from build123d import *

# Parameters (mm, degrees)
F0_W         = 12.7
F0_H         = 12.7
F1_DEPTH     = 12.7
F2_T1_DEPTH  = 6.35
F2_T3_DEPTH  = 6.35
F2_T5_DEPTH  = 6.35
F2_S9_W      = 3.175
F2_S9_H      = 3.175
F2_T10_DEPTH = 3.175
F2_S15_W     = 3.175
F2_S15_H     = 3.175
F2_T16_DEPTH = 3.175
F2_S21_W     = 3.175
F2_S21_H     = 3.175
F2_T22_DEPTH = 3.175
F2_S27_W     = 3.175
F2_S27_H     = 3.175
F2_T28_DEPTH = 3.175
F2_S33_W     = 3.175
F2_S33_H     = 3.175
F2_T34_DEPTH = 3.175
F2_S39_W     = 3.175
F2_S39_H     = 3.175
F2_T40_DEPTH = 3.175
F2_S45_W     = 3.175
F2_S45_H     = 3.175
F2_T46_DEPTH = 3.175
F2_S51_W     = 3.175
F2_S51_H     = 3.175
F2_T52_DEPTH = 3.175
F3_R         = 0.79375
F4_DEPTH     = 6.2992


# Not quite as in the source:
# - a fillet or chamfer that OpenCascade refuses, or shapes differently, is made with other operations: its cross-section is extruded or revolved along the edge and cut away or added


with BuildPart() as f1:
    # F0 (on Top) → F1 (new body)
    with BuildSketch(Plane.XY):
        Rectangle(F0_W, F0_H)
        with BuildLine():
            ThreePointArc((-2.54, 1.905), (0, 3.175), (2.54, 1.905))
            Line((2.54, 1.905), (3.96875, 0))
            Line((3.96875, 0), (2.54, -1.905))
            ThreePointArc((2.54, -1.905), (0, -3.175), (-2.54, -1.905))
            Line((-2.54, -1.905), (-3.96875, 0))
            Line((-3.96875, 0), (-2.54, 1.905))
        make_face(mode=Mode.SUBTRACT)
    extrude(amount=F1_DEPTH)

    # F2: fillet of radius 3.175 on 12 edges, made by hand

    # F2_s2 → F2_t1 (cut)
    with BuildSketch(Plane.XY.offset(3.175)):
        with BuildLine():
            ThreePointArc((6.35, -3.175), (5.4200640303, -5.4200640303), (3.175, -6.35))
            Line((3.175, -6.35), (6.35, -6.35))
            Line((6.35, -6.35), (6.35, -3.175))
        make_face()
        with BuildLine():
            ThreePointArc((6.35, 3.175), (5.4200640303, 5.4200640303), (3.175, 6.35))
            Line((3.175, 6.35), (6.35, 6.35))
            Line((6.35, 6.35), (6.35, 3.175))
        make_face()
        with BuildLine():
            ThreePointArc((-3.175, 6.35), (-5.4200640303, 5.4200640303), (-6.35, 3.175))
            Line((-6.35, 3.175), (-6.35, 6.35))
            Line((-6.35, 6.35), (-3.175, 6.35))
        make_face()
        with BuildLine():
            ThreePointArc((-6.35, -3.175), (-5.4200640303, -5.4200640303), (-3.175, -6.35))
            Line((-3.175, -6.35), (-6.35, -6.35))
            Line((-6.35, -6.35), (-6.35, -3.175))
        make_face()
    extrude(amount=F2_T1_DEPTH, mode=Mode.SUBTRACT)

    # F2_s4 → F2_t3 (cut)
    with BuildSketch(Plane.YZ.offset(-3.175)):
        with BuildLine():
            ThreePointArc((-6.35, 9.525), (-5.4200640303, 11.7700640303), (-3.175, 12.7))
            Line((-3.175, 12.7), (-6.35, 12.7))
            Line((-6.35, 12.7), (-6.35, 9.525))
        make_face()
        with BuildLine():
            ThreePointArc((-6.35, 3.175), (-5.4200640303, 0.9299359697), (-3.175, 0))
            Line((-3.175, 0), (-6.35, 0))
            Line((-6.35, 0), (-6.35, 3.175))
        make_face()
        with BuildLine():
            ThreePointArc((6.35, 3.175), (5.4200640303, 0.9299359697), (3.175, 0))
            Line((3.175, 0), (6.35, 0))
            Line((6.35, 0), (6.35, 3.175))
        make_face()
        with BuildLine():
            ThreePointArc((6.35, 9.525), (5.4200640303, 11.7700640303), (3.175, 12.7))
            Line((3.175, 12.7), (6.35, 12.7))
            Line((6.35, 12.7), (6.35, 9.525))
        make_face()
    extrude(amount=F2_T3_DEPTH, mode=Mode.SUBTRACT)

    # F2_s6 → F2_t5 (cut)
    with BuildSketch(Plane.XZ.offset(-3.175)):
        with BuildLine():
            ThreePointArc((6.35, 9.525), (5.4200640303, 11.7700640303), (3.175, 12.7))
            Line((3.175, 12.7), (6.35, 12.7))
            Line((6.35, 12.7), (6.35, 9.525))
        make_face()
        with BuildLine():
            ThreePointArc((6.35, 3.175), (5.4200640303, 0.9299359697), (3.175, 0))
            Line((3.175, 0), (6.35, 0))
            Line((6.35, 0), (6.35, 3.175))
        make_face()
        with BuildLine():
            ThreePointArc((-6.35, 3.175), (-5.4200640303, 0.9299359697), (-3.175, 0))
            Line((-3.175, 0), (-6.35, 0))
            Line((-6.35, 0), (-6.35, 3.175))
        make_face()
        with BuildLine():
            ThreePointArc((-6.35, 9.525), (-5.4200640303, 11.7700640303), (-3.175, 12.7))
            Line((-3.175, 12.7), (-6.35, 12.7))
            Line((-6.35, 12.7), (-6.35, 9.525))
        make_face()
    extrude(amount=F2_T5_DEPTH, mode=Mode.SUBTRACT)


with BuildPart() as f2_tool8:
    # F2_s9 → F2_t10 (new body)
    with BuildSketch(Plane.YZ.offset(3.175)):
        with Locations((-4.7625, 1.5875)):
            Rectangle(F2_S9_W, F2_S9_H)
    extrude(amount=F2_T10_DEPTH)

    # F2_s11 → F2_t12 (revolve, cut)
    with BuildSketch(Plane(origin=(3.175, -3.175, 3.175), x_dir=(0, 0.7071067812, 0.7071067812), z_dir=(0, 0.7071067812, -0.7071067812))):
        with BuildLine():
            ThreePointArc((0, -3.175), (3.175, 0), (0, 3.175))
            Line((0, 3.175), (0, -3.175))
        make_face()
    revolve(axis=Axis((3.175, -3.175, 3.175), (1, 0, 0)), mode=Mode.SUBTRACT)


with BuildPart() as f1_1:
    add(f1.part)

    # F2_t7: cut F2_tool8
    add(f2_tool8.part, mode=Mode.SUBTRACT)


with BuildPart() as f2_tool14:
    # F2_s15 → F2_t16 (new body)
    with BuildSketch(Plane.YZ.offset(3.175)):
        with Locations((-4.7625, 11.1125)):
            Rectangle(F2_S15_W, F2_S15_H)
    extrude(amount=F2_T16_DEPTH)

    # F2_s17 → F2_t18 (revolve, cut)
    with BuildSketch(Plane(origin=(3.175, -3.175, 9.525), x_dir=(0, 0.7071067812, -0.7071067812), z_dir=(0, -0.7071067812, -0.7071067812))):
        with BuildLine():
            ThreePointArc((0, -3.175), (3.175, 0), (0, 3.175))
            Line((0, 3.175), (0, -3.175))
        make_face()
    revolve(axis=Axis((3.175, -3.175, 9.525), (1, 0, 0)), mode=Mode.SUBTRACT)


with BuildPart() as f1_2:
    add(f1_1.part)

    # F2_t13: cut F2_tool14
    add(f2_tool14.part, mode=Mode.SUBTRACT)


with BuildPart() as f2_tool20:
    # F2_s21 → F2_t22 (new body)
    with BuildSketch(Plane.XY.offset(9.525)):
        with Locations((-4.7625, -4.7625)):
            Rectangle(F2_S21_W, F2_S21_H)
    extrude(amount=F2_T22_DEPTH)

    # F2_s23 → F2_t24 (revolve, cut)
    with BuildSketch(Plane(origin=(-3.175, -3.175, 9.525), x_dir=(0.7071067812, 0.7071067812, 0), z_dir=(0.7071067812, -0.7071067812, 0))):
        with BuildLine():
            ThreePointArc((0, -3.175), (3.175, 0), (0, 3.175))
            Line((0, 3.175), (0, -3.175))
        make_face()
    revolve(axis=Axis((-3.175, -3.175, 9.525), (0, 0, 1)), mode=Mode.SUBTRACT)


with BuildPart() as f1_3:
    add(f1_2.part)

    # F2_t19: cut F2_tool20
    add(f2_tool20.part, mode=Mode.SUBTRACT)


with BuildPart() as f2_tool26:
    # F2_s27 → F2_t28 (new body)
    with BuildSketch(Plane.YZ.offset(3.175)):
        with Locations((4.7625, 11.1125)):
            Rectangle(F2_S27_W, F2_S27_H)
    extrude(amount=F2_T28_DEPTH)

    # F2_s29 → F2_t30 (revolve, cut)
    with BuildSketch(Plane(origin=(3.175, 3.175, 9.525), x_dir=(0, -0.7071067812, -0.7071067812), z_dir=(0, -0.7071067812, 0.7071067812))):
        with BuildLine():
            ThreePointArc((0, -3.175), (3.175, 0), (0, 3.175))
            Line((0, 3.175), (0, -3.175))
        make_face()
    revolve(axis=Axis((3.175, 3.175, 9.525), (1, 0, 0)), mode=Mode.SUBTRACT)


with BuildPart() as f1_4:
    add(f1_3.part)

    # F2_t25: cut F2_tool26
    add(f2_tool26.part, mode=Mode.SUBTRACT)


with BuildPart() as f2_tool32:
    # F2_s33 → F2_t34 (new body)
    with BuildSketch(Plane.YZ.offset(3.175)):
        with Locations((4.7625, 1.5875)):
            Rectangle(F2_S33_W, F2_S33_H)
    extrude(amount=F2_T34_DEPTH)

    # F2_s35 → F2_t36 (revolve, cut)
    with BuildSketch(Plane(origin=(3.175, 3.175, 3.175), x_dir=(0, -0.7071067812, 0.7071067812), z_dir=(0, 0.7071067812, 0.7071067812))):
        with BuildLine():
            ThreePointArc((0, -3.175), (3.175, 0), (0, 3.175))
            Line((0, 3.175), (0, -3.175))
        make_face()
    revolve(axis=Axis((3.175, 3.175, 3.175), (1, 0, 0)), mode=Mode.SUBTRACT)


with BuildPart() as f1_5:
    add(f1_4.part)

    # F2_t31: cut F2_tool32
    add(f2_tool32.part, mode=Mode.SUBTRACT)


with BuildPart() as f2_tool38:
    # F2_s39 → F2_t40 (new body)
    with BuildSketch(Plane.YZ.offset(-3.175)):
        with Locations((-4.7625, 1.5875)):
            Rectangle(F2_S39_W, F2_S39_H)
    extrude(amount=-F2_T40_DEPTH)

    # F2_s41 → F2_t42 (revolve, cut)
    with BuildSketch(Plane(origin=(-3.175, -3.175, 3.175), x_dir=(0, 0.7071067812, 0.7071067812), z_dir=(0, -0.7071067812, 0.7071067812))):
        with BuildLine():
            ThreePointArc((0, -3.175), (3.175, 0), (0, 3.175))
            Line((0, 3.175), (0, -3.175))
        make_face()
    revolve(axis=Axis((-3.175, -3.175, 3.175), (-1, 0, 0)), mode=Mode.SUBTRACT)


with BuildPart() as f1_6:
    add(f1_5.part)

    # F2_t37: cut F2_tool38
    add(f2_tool38.part, mode=Mode.SUBTRACT)


with BuildPart() as f2_tool44:
    # F2_s45 → F2_t46 (new body)
    with BuildSketch(Plane.XZ.offset(-3.175)):
        with Locations((-4.7625, 1.5875)):
            Rectangle(F2_S45_W, F2_S45_H)
    extrude(amount=-F2_T46_DEPTH)

    # F2_s47 → F2_t48 (revolve, cut)
    with BuildSketch(Plane(origin=(-3.175, 3.175, 3.175), x_dir=(0.7071067812, 0, 0.7071067812), z_dir=(-0.7071067812, 0, 0.7071067812))):
        with BuildLine():
            ThreePointArc((0, -3.175), (3.175, 0), (0, 3.175))
            Line((0, 3.175), (0, -3.175))
        make_face()
    revolve(axis=Axis((-3.175, 3.175, 3.175), (0, 1, 0)), mode=Mode.SUBTRACT)


with BuildPart() as f1_7:
    add(f1_6.part)

    # F2_t43: cut F2_tool44
    add(f2_tool44.part, mode=Mode.SUBTRACT)


with BuildPart() as f2_tool50:
    # F2_s51 → F2_t52 (new body)
    with BuildSketch(Plane.XZ.offset(-3.175)):
        with Locations((-4.7625, 11.1125)):
            Rectangle(F2_S51_W, F2_S51_H)
    extrude(amount=-F2_T52_DEPTH)

    # F2_s53 → F2_t54 (revolve, cut)
    with BuildSketch(Plane(origin=(-3.175, 3.175, 9.525), x_dir=(0.7071067812, 0, -0.7071067812), z_dir=(0.7071067812, 0, 0.7071067812))):
        with BuildLine():
            ThreePointArc((0, -3.175), (3.175, 0), (0, 3.175))
            Line((0, 3.175), (0, -3.175))
        make_face()
    revolve(axis=Axis((-3.175, 3.175, 9.525), (0, 1, 0)), mode=Mode.SUBTRACT)


with BuildPart() as f1_8:
    add(f1_7.part)

    # F2_t49: cut F2_tool50
    add(f2_tool50.part, mode=Mode.SUBTRACT)

    # F3 (on face) → F4 (cut)
    with BuildSketch(Plane.YZ.offset(6.35)):
        with Locations((0, 6.35)):
            Circle(F3_R)
    extrude(amount=-F4_DEPTH, mode=Mode.SUBTRACT)


solid = f1_8.part
Here's how the part is built. I have some questions about the finished solid (model axes, mm). A direction names the side the tool comes from. Coordinates: 2 decimals unless noted, no trailing zeros. Loops run counter-clockwise (first coordinate to the right, second up) from the corner with the lowest first, then second, coordinate; pieces in that order, holes last.
1. Imagine slicing it at D-D, the plane y = -5.25. Please give me the cut outline in (x, z) (3 decimals).
2. If we mould it in two halves opening along X, with no side actions, what happens to faces 3 (the flat face through (-2, 3, 12.7)), 4 (the flat face through (-3.24, -0.97, 6.26)), 5 (the cylindrical face through (5.44, 0.04, 0.95))? For each: pulls with the +X half, pulls with the -X half, needs draft (parallel to the pull), parting line crosses it, or undercut.
3. For faces 1 (the flat face through (3.264, -0.939, 6.261)), 2 (the cylindrical face through (-0.04, 5.44, 11.75)), which set-ups out of +Z, -Z, +X, -X, +Y, -Y let a thin tool reach every point of the face, with its end or its side?
4. For P1, Ø1.5, axis at y = 3, z = 2, coming from the -X side, with a flat end and sliding along its axis, tell me the tip position at first contact or that it passes through.
5. Imagine slicing it at B-B, the plane x = 2.75. Please give me the cut outline in (y, z) (3 decimals).
6. I need wall thicknesses on L1, parallel to X at y = 2, z = 7.75; L2, parallel to Y at x = 5.3, z = 6.35; L3, parallel to Y at x = 1.5, z = 10.75. Which ranges of each line are inside material? Lowest first, please.
7. Imagine slicing it at A-A, the plane z = 5.25. Please give me the cut outline in (x, y) (3 decimals), and give its area (3 significant figures).
Taken from the geometry:
1. outline: (-5.578, 3.175) arc R2.403 ccw to (-3.175, 0.772) - (3.175, 0.772) arc R2.403 ccw to (5.578, 3.175) - (5.578, 9.525) arc R2.403 ccw to (3.175, 11.928) - (-3.175, 11.928) arc R2.403 ccw to (-5.578, 9.525) - close
2. face 3: needs draft
2. face 4: undercut
2. face 5: pulls with the +X half
3. face 1: +Z, -Z
3. face 2: +Z, +X, -X, +Y
4. P1: stops at x = -6.32
5. outline: (-6.35, 3.175) arc R3.175 ccw to (-3.175, 0) - (-1.625, 0) - (-1.625, 12.7) - (-3.175, 12.7) arc R3.175 ccw to (-6.35, 9.525) - close; (1.625, 0) - (3.175, 0) arc R3.175 ccw to (6.35, 3.175) - (6.35, 9.525) arc R3.175 ccw to (3.175, 12.7) - (1.625, 12.7) - close
6. L1: x = -6.35 to -2.47, 2.47 to 6.35
6. L2: y = -5.53 to -0.79, 0.79 to 5.53
6. L3: y = -6.1 to -2.8, 2.8 to 6.1
7. outline: (-6.35, -3.175) arc R3.175 ccw to (-3.175, -6.35) - (3.175, -6.35) arc R3.175 ccw to (6.35, -3.175) - (6.35, 3.175) arc R3.175 ccw to (3.175, 6.35) - (-3.175, 6.35) arc R3.175 ccw to (-6.35, 3.175) - close; hole (-3.969, 0) - (-2.54, -1.905) arc R3.175 ccw to (2.54, -1.905) - (3.969, 0) - (2.54, 1.905) arc R3.175 ccw to (-2.54, 1.905) - close
7. area: 119 mm2
